```python
from build123d import *

# Parameters (mm, degrees)
SKETCH3_R           = 46
BOSS_EXTRUDE1_DEPTH = 3
SKETCH2_R           = 28
CUT_EXTRUDE1_DEPTH  = 172.350517945
SKETCH5_R           = 8
CUT_EXTRUDE7_DEPTH  = 170.917627149
CIRPATTERN2_COUNT   = 4
SKETCH7_W           = 16
SKETCH7_H           = 6
CUT_EXTRUDE8_DEPTH  = 172.350517993


with BuildPart() as part:
    # Sketch1 → Revolve1 (revolve)
    with BuildSketch(Plane.XY, mode=Mode.PRIVATE) as revolve1_sk:
        with BuildLine():
            Line((0, 0), (80, 0))
            Line((80, 0), (80, 54))
            ThreePointArc((80, 54), (79.414213562, 55.414213562), (78, 56))
            Line((78, 56), (28.292682927, 56))
            Line((28.292682927, 56), (22, 56))
            Line((22, 56), (22, 98))
            ThreePointArc((22, 98), (22.585786438, 99.414213562), (24, 100))
            Line((24, 100), (38, 100))
            ThreePointArc((38, 100), (39.414213562, 100.585786438), (40, 102))
            Line((40, 102), (40, 104))
            ThreePointArc((40, 104), (39.414213562, 105.414213562), (38, 106))
            Line((38, 106), (0, 106))
            Line((0, 106), (0, 0))
        make_face()
    revolve(revolve1_sk.sketch.rotate(Axis((0, 0, 0), (1, 0, 0)), 90), axis=Axis((0, 0, 0), (1, 0, 0)))

    # Sketch3 → Boss-Extrude1 (add)
    with BuildSketch(Plane.ZY):
        with Locations(Location((0, 0, 0), (0, 0, 180))):
            Circle(SKETCH3_R)
    extrude(amount=BOSS_EXTRUDE1_DEPTH)

    # Sketch2 → Cut-Extrude1 (cut, through all)
    with BuildSketch(Plane(origin=(80, 0, 0), x_dir=(0, 0, -1), z_dir=(1, 0, 0))):
        Circle(SKETCH2_R)
    extrude(amount=-CUT_EXTRUDE1_DEPTH, mode=Mode.SUBTRACT)

    # Sketch5 → Cut-Extrude7 (cut, through all)
    with BuildSketch(Plane.ZY):
        with Locations((0, 80)):
            Circle(SKETCH5_R)
    cut_extrude7 = extrude(amount=-CUT_EXTRUDE7_DEPTH, mode=Mode.SUBTRACT)

    # CirPattern2: Cut-Extrude7 ×4 about axis
    cirpattern2_axis = Axis((0, 0, 0), (1, 0, 0))
    for i in range(1, CIRPATTERN2_COUNT):
        add(cut_extrude7.rotate(cirpattern2_axis, i * 360 / CIRPATTERN2_COUNT), mode=Mode.SUBTRACT)

    # Sketch7 → Cut-Extrude8 (cut, through all)
    with BuildSketch(Plane.ZY.offset(3)):
        with Locations((0, 30)):
            Rectangle(SKETCH7_W, SKETCH7_H)
    extrude(amount=-CUT_EXTRUDE8_DEPTH, mode=Mode.SUBTRACT)


solid = part.part
```
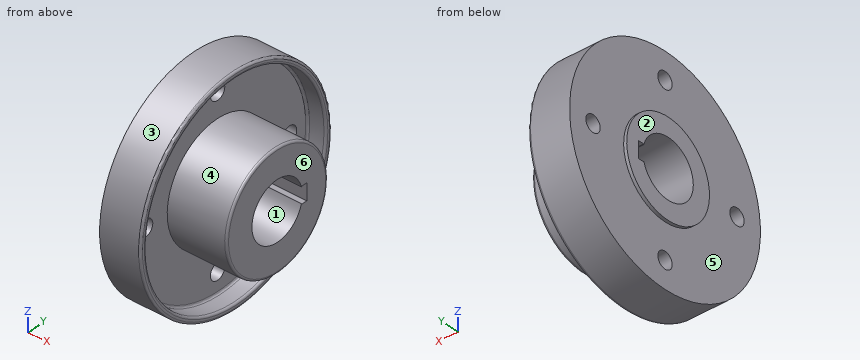
Can you work these out from the model? Positions are in its coordinate system, mm. Face numbers are marked on the shaded views. A direction names the side the tool comes from. Coordinates: 2 decimals unless noted, no trailing zeros. Loops run counter-clockwise (first coordinate to the right, second up) from the corner with the lowest first, then second, coordinate; pieces in that order, holes last.
Item 1: Which directions (+Z, -Z, +X, -X, +Y, -Y) give clear straight access to the entire face, cutting with the end or side of a thin tool? Please do the marked faces 4, 5 and 6.
Answers below:
face 4: +X
face 5: -X
face 6: +Z, -Z, +X, +Y, -Y
Item 2: Suppose I cut it at C-C (y = 0). State how many separate pieces and enclosed holes the cut face has, then the cut area to 3 significant figures.
Answers below:
separate pieces: 4
enclosed holes: 0
area: 6,300 mm2
Item 3: Suppose I cut it at A-A (x = 29). Please give me the cut outline in (y, z).
Answers below:
outline: circle Ø212 at (0, 0); circle Ø112 at (0, 0); hole circle Ø200 at (0, 0); hole (27, -8) - (33, -8) - (33, 8) - (27, 8) - (27, 7.42) arc R28 ccw (long way) to (27, -7.42) - close
Item 4: If we mould it in two halves opening along Y, with no side actions, what happens to the marked faces 1, 2 and 3? For each: released by +Y, released by -Y, zero draft, split by the parting line, or undercut.
Answers below:
face 1: undercut
face 2: zero draft
face 3: split by the parting line
Item 5: I'm going to push flat-ended pins straight in: pin 1 (1.8 mm diameter, centred on x = 27, y = 30.5, fed in from -Z); pin 2 (6 mm diameter, centred on x = 33.5, z = -39, fed in from -Y); pin 3 (10 mm diameter, centred on y = -73.5, z = -37.5, fed in from +X). Where does each tip first touch, or does it pass through?
Answers below:
pin 1: stops at z = -101.78
pin 2: stops at y = -99.7
pin 3: stops at x = 22
Item 6: Please list where these lines run through material, in increasing order: L1, parallel to Y at x = 36, z = -37; L2, parallel to Z at x = 31, y = -16.5; L3, parallel to Z at x = 14, y = -80.
Answers below:
L1: y = -99.33 to -92.9, -42.04 to 42.04, 92.9 to 99.33
L2: z = -104.71 to -98.63, -53.51 to -22.62, 22.62 to 53.51, 98.63 to 104.71
L3: z = -69.54 to -8, 8 to 69.54
Item 7: Suppose I cut it at B-B (x = 59). Please give me the cut outline in (y, z).
Answers below:
outline: circle Ø112 at (0, 0); hole (27, -8) - (33, -8) - (33, 8) - (27, 8) - (27, 7.42) arc R28 ccw (long way) to (27, -7.42) - close
